Can you work these out from the model? Positions are in its coordinate system, mm. Face numbers are marked on the shaded views. A direction names the side the tool comes from. Round coordinates to 2 decimals unless told otherwise and drop trailing zeros. Loops run counter-clockwise (first coordinate to the right, second up) from the corner with the lowest first, then second, coordinate; pieces in that order, holes last. Notation, with made-up numbers: (-22.5, 89) -> (20.5, 89) arc R26 ccw to (20.5, 122) -> close; hole circle Ø9 at (71.5, 49). An arc over 180 degrees is marked (long way). Answer as a JSON object with one key per item and string values.
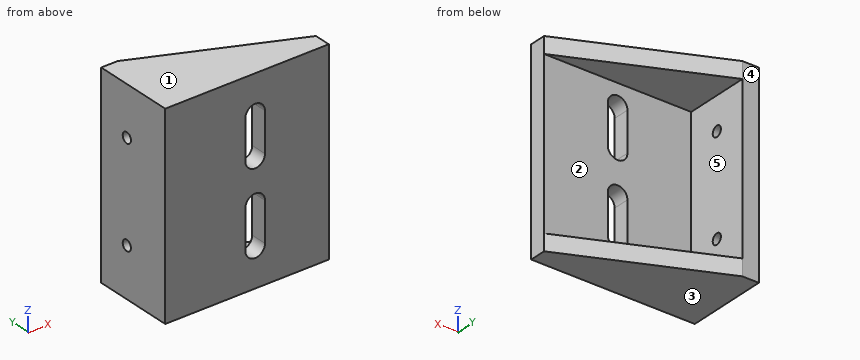
```python
from build123d import *

# Parameters (mm, degrees)
BOSS_EXTRUDE1_DEPTH = 60
BOSS_EXTRUDE2_DEPTH = 5
BOSS_EXTRUDE3_DEPTH = 5
SKETCH4_R           = 1.6
CUT_EXTRUDE1_DEPTH  = 5
CUT_EXTRUDE2_DEPTH  = 5


with BuildPart() as part:
    # Sketch1 → Boss-Extrude1 (new body)
    with BuildSketch(Plane.XY):
        Polygon((0, 0), (-50, 0), (-50, 25), (-45, 25), (-45, 5), (0, 5), align=None)
    extrude(amount=BOSS_EXTRUDE1_DEPTH)

    # Sketch2 → Boss-Extrude2 (add)
    with BuildSketch(Plane.XY.offset(60)):
        Polygon((-45, 25), (0, 5), (-45, 5), align=None)
    extrude(amount=-BOSS_EXTRUDE2_DEPTH)

    # Sketch3 → Boss-Extrude3 (add)
    with BuildSketch(Plane(origin=(0, 0, 0), x_dir=(-1, 0, 0), z_dir=(0, 0, -1))):
        Polygon((45, 25), (0, 5), (45, 5), align=None)
    extrude(amount=-BOSS_EXTRUDE3_DEPTH)

    # Sketch4 → Cut-Extrude1 (cut)
    with BuildSketch(Plane(origin=(-45, 0, 0), x_dir=(0, 0, -1), z_dir=(1, 0, 0))):
        with Locations((-45, 15)):
            Circle(SKETCH4_R)
        with Locations((-15, 15)):
            Circle(SKETCH4_R)
    extrude(amount=-CUT_EXTRUDE1_DEPTH, mode=Mode.SUBTRACT)

    # Sketch5 → Cut-Extrude2 (cut)
    with BuildSketch(Plane(origin=(0, 5, 0), x_dir=(1, 0, 0), z_dir=(0, 1, 0))):
        with BuildLine():
            Line((-25.5, -23.5), (-25.5, -11.5))
            ThreePointArc((-25.5, -11.5), (-22.5, -8.5), (-19.5, -11.5))
            Line((-19.5, -11.5), (-19.5, -23.5))
            ThreePointArc((-19.5, -23.5), (-22.5, -26.5), (-25.5, -23.5))
        make_face()
        with BuildLine():
            Line((-19.5, -48.5), (-19.5, -36.5))
            ThreePointArc((-19.5, -36.5), (-22.5, -33.5), (-25.5, -36.5))
            Line((-25.5, -36.5), (-25.5, -48.5))
            ThreePointArc((-25.5, -48.5), (-22.5, -51.5), (-19.5, -48.5))
        make_face()
    extrude(amount=-CUT_EXTRUDE2_DEPTH, mode=Mode.SUBTRACT)


solid = part.part
```
Q1. On a 3-axis mill with a long thin cutter (end or side, diameter ignored), from which of +Z, -Z, +X, -X, +Y, -Y can I reach the whole of each face in a straight line? I mean the marked faces 4 and 5. Say none if no direction works.
Determined:
{"face 4": "+Z, -Z, +X, -X, +Y", "face 5": "+X, +Y"}
Q2. If I drill on L1, parallel to Y at x = -47, z = 15; L2, parallel to Z at x = -33, y = 17; L3, parallel to Y at x = -33, z = 15.5, over which ranges is the centre line in solid material (lowest first)? Write a range as [from, to].
Determined:
{"L1": "[0, 13.4], [16.6, 25]", "L2": "[0, 5], [55, 60]", "L3": "[0, 5]"}
Q3. I want a section at B-B, the plane y = 15. Write out the boundary of the cut face in (x, z).
Determined:
{"outline": "(-50, 0) -> (-22.5, 0) -> (-22.5, 5) -> (-45, 5) -> (-45, 13.4) -> (-50, 13.4) -> close; (-50, 16.6) -> (-45, 16.6) -> (-45, 43.4) -> (-50, 43.4) -> close; (-50, 46.6) -> (-45, 46.6) -> (-45, 55) -> (-22.5, 55) -> (-22.5, 60) -> (-50, 60) -> close"}
Q4. I'm going to push flat-ended pins straight in: pin 1 (5 mm diameter, centred on y = 15, z = 45, fed in from +X); pin 2 (1 mm diameter, centred on x = -15.5, z = 40.5, fed in from +Y); pin 3 (3 mm diameter, centred on x = -39, z = 38.5, fed in from -Y); pin 4 (1.9 mm diameter, centred on y = 15, z = 15, fed in from +X). Where does each tip first touch, or does it pass through?
Determined:
{"pin 1": "x = -45", "pin 2": "y = 5", "pin 3": "y = 0", "pin 4": "through"}
Q5. I want a section at D-D, the plane y = 3. Write out the boundary of the cut face in (x, z), then the cut area to 3 significant figures.
Determined:
{"outline": "(-50, 0) -> (0, 0) -> (0, 60) -> (-50, 60) -> close; hole (-25.5, 11.5) arc R3 ccw to (-19.5, 11.5) -> (-19.5, 23.5) arc R3 ccw to (-25.5, 23.5) -> close; hole (-25.5, 36.5) arc R3 ccw to (-19.5, 36.5) -> (-19.5, 48.5) arc R3 ccw to (-25.5, 48.5) -> close", "area": "2,800 mm²"}
Q6. I want a section at C-C, the plane z = 15. Write out the boundary of the cut face in (x, y).
Determined:
{"outline": "(-50, 0) -> (-25.5, 0) -> (-25.5, 5) -> (-45, 5) -> (-45, 13.4) -> (-50, 13.4) -> close; (-50, 16.6) -> (-45, 16.6) -> (-45, 25) -> (-50, 25) -> close; (-19.5, 0) -> (0, 0) -> (0, 5) -> (-19.5, 5) -> close"}
Q7. We'd pull the mould along Z, two halves only. Please class the marked faces 1, 2 and 3: pulls with the +Z half, pulls with the -Z half, needs draft (parallel to the pull), parting line crosses it, or undercut.
Determined:
{"face 1": "pulls with the +Z half", "face 2": "undercut", "face 3": "pulls with the -Z half"}
Q8. I want a section at A-A, the plane x = -22.5. Write out the boundary of the cut face in (y, z), then the cut area to 3 significant figures.
Determined:
{"outline": "(0, 0) -> (15, 0) -> (15, 5) -> (5, 5) -> (5, 8.5) -> (0, 8.5) -> close; (0, 26.5) -> (5, 26.5) -> (5, 33.5) -> (0, 33.5) -> close; (0, 51.5) -> (5, 51.5) -> (5, 55) -> (15, 55) -> (15, 60) -> (0, 60) -> close", "area": "220 mm²"}
